Build history of the part. All positions in model axes, mm. A direction names the side the tool comes from. Coordinates: 2 decimals unless noted, no trailing zeros. Order: outer loops, then holes, each group sorted by start corner. A loop starts at its lowest first (then second) coordinate and runs counter-clockwise, first axis right, second up. Notation, with made-up numbers: (36.25, 67) - (95.25, 67) arc R27 ccw to (95.25, 87) - close; hole circle Ø3 at (55, 4). An arc over 180 degrees is marked (long way). Answer as CSV lines item,"result". Start each with the question number.
from build123d import *

# Parameters (mm, degrees)
SKETCH1_W                 = 12.5
SKETCH1_H                 = 11.5
BOSS_EXTRUDE1_DEPTH       = 109
SKETCH2_W                 = 24
SKETCH2_H                 = 20
BOSS_EXTRUDE2_DEPTH       = 3.5
F_2_5MM_DOWEL_HOLE1_D     = 3.2
F_2_5MM_DOWEL_HOLE1_DEPTH = 6.5
F_2_5MM_DOWEL_HOLE1_TIP   = 0.96137699
SKETCH5_W                 = 8
SKETCH5_H                 = 2.5
CUT_EXTRUDE1_DEPTH        = 117.757226757
FILLET1_R                 = 4
CHAMFER1_SIZE             = 0.5
FILLET2_R                 = 1


with BuildPart() as part:
    # Sketch1 → Boss-Extrude1 (new body)
    with BuildSketch(Plane.XY):
        Polygon((-37.25, 0), (-37.25, 11.5), (-37.25, 20), (-43, 20), (-43, 0), align=None)
        with Locations((-31, 5.75)):
            Rectangle(SKETCH1_W, SKETCH1_H)
        Polygon((-24.75, 20), (-24.75, 11.5), (-24.75, 0), (-19, 0), (-19, 20), align=None)
    extrude(amount=BOSS_EXTRUDE1_DEPTH)

    # Sketch2 → Boss-Extrude2 (add)
    with BuildSketch(Plane.XY.offset(109)):
        with Locations((-31, 10)):
            Rectangle(SKETCH2_W, SKETCH2_H)
    extrude(amount=BOSS_EXTRUDE2_DEPTH)

    # Ø2.5mm Dowel Hole1
    with Locations(Plane(origin=(0, 0, 0), x_dir=(-1, 0, 0), z_dir=(0, 0, -1))):
        with Locations((36, 5.6), (26, 5.6)):
            Hole(F_2_5MM_DOWEL_HOLE1_D / 2, depth=F_2_5MM_DOWEL_HOLE1_DEPTH)
            with Locations((0, 0, -(F_2_5MM_DOWEL_HOLE1_DEPTH + F_2_5MM_DOWEL_HOLE1_TIP / 2))):  # 118° drill point
                Cone(0, F_2_5MM_DOWEL_HOLE1_D / 2, F_2_5MM_DOWEL_HOLE1_TIP, mode=Mode.SUBTRACT)

    # Sketch5 → Cut-Extrude1 (cut, through all)
    with BuildSketch(Plane(origin=(-19, 0, 0), x_dir=(0, 0, -1), z_dir=(1, 0, 0))):
        with Locations((-89.5, 4)):
            Rectangle(SKETCH5_W, SKETCH5_H)
        with Locations((-19.5, 4)):
            Rectangle(SKETCH5_W, SKETCH5_H)
    extrude(amount=-CUT_EXTRUDE1_DEPTH, mode=Mode.SUBTRACT)

    # Fillet1
    fillet1_edges = [part.edges().sort_by_distance(p)[0] for p in [
        (-43, 5.25, 89.5),
        (-19, 5.25, 89.5),
        (-43, 5.25, 19.5),
        (-19, 5.25, 19.5),
    ]]
    fillet(fillet1_edges, radius=FILLET1_R)

    # Chamfer1
    chamfer1_edges = [part.edges().sort_by_distance(p)[0] for p in [
        (-37.6, 5.6, 0),
        (-27.6, 5.6, 0),
    ]]
    chamfer(chamfer1_edges, length=CHAMFER1_SIZE)

    # Fillet2
    fillet2_edges = [part.edges().sort_by_distance(p)[0] for p in [
        (-37.25, 11.5, 54.5),
        (-24.75, 11.5, 54.5),
    ]]
    fillet(fillet2_edges, radius=FILLET2_R)


solid = part.part
(1) Probe L1, parallel to X at y = 5.6, z = 4.9; L2, parallel to Z at x = -33.75, y = 3.75; L3, parallel to Y at x = -36, z = 3.8. List the from-to ranges inside material, lowest first. Write a range as [from, to].
(2) Which spindle directions (+Z, -Z, +X, -X, +Y, -Y) get a long thin tool onto all of the face, cutting with end or side? Do faces 1 (the cylindrical face through (-20.203, 6.391, 89.444)), 2 (the flat face through (-31, 16, 109)), 3 (the flat face through (-31, 5.25, 90)), 4 (the cylindrical face through (-37.18, 6.68, 3.54)), 5 (the cylindrical face through (-41.859, 6.453, 19.556)). Say none if no direction does.
(3) Band-saw the part on C-C on z = 75.5. List the corners of the cut face in (x, y).
(4) Band-saw the part on D-D on x = -21.5. List the corners of the cut face in (y, z), plus the area to 3 significant figures.
(5) Band-saw the part on B-B on y = 18.5. List the corners of the cut face in (x, z).
(6) Drop flat-ended pins along their axis: pin 1 Ø4 at (x, y) = (-26, 5.6) entering from -Z; pin 2 Ø7 at (x, y) = (-29, 16.5) entering from -Z; pin 3 Ø9 at (x, z) = (-29.5, 18.5) entering from +Y. Give the stop position or say it passes through.
(7) Pull direction Y, two halves, no side cores. Call faces 6 (the flat face through (-31, 2.75, 90)), 7 (the flat face through (-31, 5.25, 20)), 8 (the flat face through (-31, 8, 0)), 9 (the flat face through (-39, 20, 55)): +Y half, -Y half, draft (parallel to the pull), parting line (faces both ways), or undercut.
(8) Band-saw the part on A-A on x = -29.5. List the corners of the cut face in (y, z), plus the area to 3 significant figures.
Filled in:
1,L1,"x = [-43, -37.6], [-34.4, -27.6], [-24.4, -19]"
1,L2,"z = [0, 15.5], [23.5, 85.5], [93.5, 112.5]"
1,L3,"y = [0, 4], [7.2, 11.5]"
2,face 1,"+X"
2,face 2,"-Z, +Y"
2,face 3,"+X, -X"
2,face 4,"-Z"
2,face 5,"-X"
3,outline,"(-43, 0) - (-19, 0) - (-19, 20) - (-24.75, 20) - (-24.75, 12.5) arc R1 cw to (-25.75, 11.5) - (-36.25, 11.5) arc R1 cw to (-37.25, 12.5) - (-37.25, 20) - (-43, 20) - close"
4,outline,"(0, 0) - (20, 0) - (20, 112.5) - (0, 112.5) - close; hole (2.75, 15.5) - (5.54, 15.5) - (5.54, 23.5) - (2.75, 23.5) - close; hole (2.75, 85.5) - (5.54, 85.5) - (5.54, 93.5) - (2.75, 93.5) - close"
4,area,"2,210 mm^2"
5,outline,"(-43, 0) - (-37.25, 0) - (-37.25, 109) - (-24.75, 109) - (-24.75, 0) - (-19, 0) - (-19, 112.5) - (-43, 112.5) - close"
6,pin 1,"stops at z = 0.1"
6,pin 2,"stops at z = 109"
6,pin 3,"stops at y = 11.84"
7,face 6,"undercut"
7,face 7,"undercut"
7,face 8,"draft"
7,face 9,"+Y half"
8,outline,"(0, 0) - (11.5, 0) - (11.5, 109) - (20, 109) - (20, 112.5) - (0, 112.5) - close; hole (2.75, 15.5) - (5.25, 15.5) - (5.25, 23.5) - (2.75, 23.5) - close; hole (2.75, 85.5) - (5.25, 85.5) - (5.25, 93.5) - (2.75, 93.5) - close"
8,area,"1,280 mm^2"
